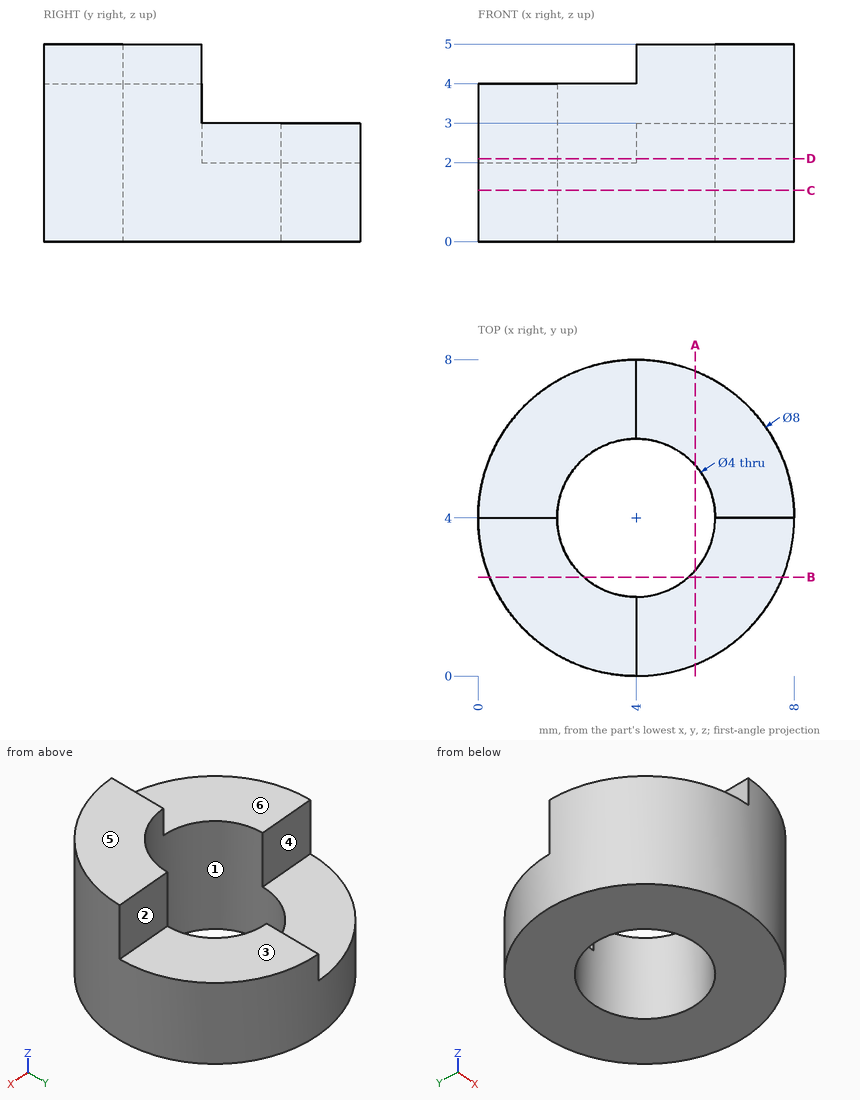
Print and shaded views of the part. All mm, measured from the part's lowest x, y and z. A direction names the side the tool comes from. Coordinates: 2 decimals unless noted, no trailing zeros. Order: outer loops, then holes, each group sorted by start corner. A loop starts at its lowest first (then second) coordinate and runs counter-clockwise, first axis right, second up.
Item 1: Saw through at C-C on z = 1.3. List the corners of the cut face in (x, y).
Filled in:
outline: circle Ø8 at (4, 4); hole circle Ø4 at (4, 4)
Item 2: Saw through at D-D on z = 2.1. List the corners of the cut face in (x, y).
Filled in:
outline: (0, 4) arc R4 ccw (long way) to (4, 8) - (4, 6) arc R2 cw (long way) to (2, 4) - close
Item 3: Tool access for the marked faces 4, 5 and 6: list every direction of +Z, -Z, +X, -X, +Y, -Y with a clear straight run to the whole face (end or side of a thin tool).
Filled in:
face 4: +Z, -X, +Y
face 5: +Z, +X, -X, +Y, -Y
face 6: +Z, -X, +Y, -Y
Item 4: Drill centre lines: L1, parallel to X at y = 4, z = 1.1; L2, parallel to X at y = 3.25, z = 2.4. Where is each one in solid material? Low to high.
Filled in:
L1: x = 0 to 2, 6 to 8
L2: x = 0.07 to 2.15, 5.85 to 7.93
Item 5: Drop flat-ended pins along their axis: pin 1 Ø1.2 at (x, y) = (1.5, 3) entering from +Z; pin 2 Ø3 at (x, y) = (6, 6.5) entering from +Z; pin 3 Ø2 at (y, z) = (2, 1) entering from +X. Give the stop position or say it passes through.
Filled in:
pin 1: stops at z = 4
pin 2: stops at z = 3
pin 3: stops at x = 7.87
Item 6: Mould opens along Y. For the marked faces 1, 2 and 3 say: released by +Y, released by -Y, zero draft, split by the parting line, or undercut.
Filled in:
face 1: undercut
face 2: released by +Y
face 3: zero draft
Item 7: Saw through at A-A on x = 5.5. List the corners of the cut face in (y, z).
Filled in:
outline: (0.29, 0) - (2.68, 0) - (2.68, 5) - (0.29, 5) - close; (5.32, 0) - (7.71, 0) - (7.71, 3) - (5.32, 3) - close
Item 8: Saw through at B-B on y = 2.5. List the corners of the cut face in (x, z).
Filled in:
outline: (0.29, 0) - (2.68, 0) - (2.68, 4) - (0.29, 4) - close; (5.32, 0) - (7.71, 0) - (7.71, 5) - (5.32, 5) - close
